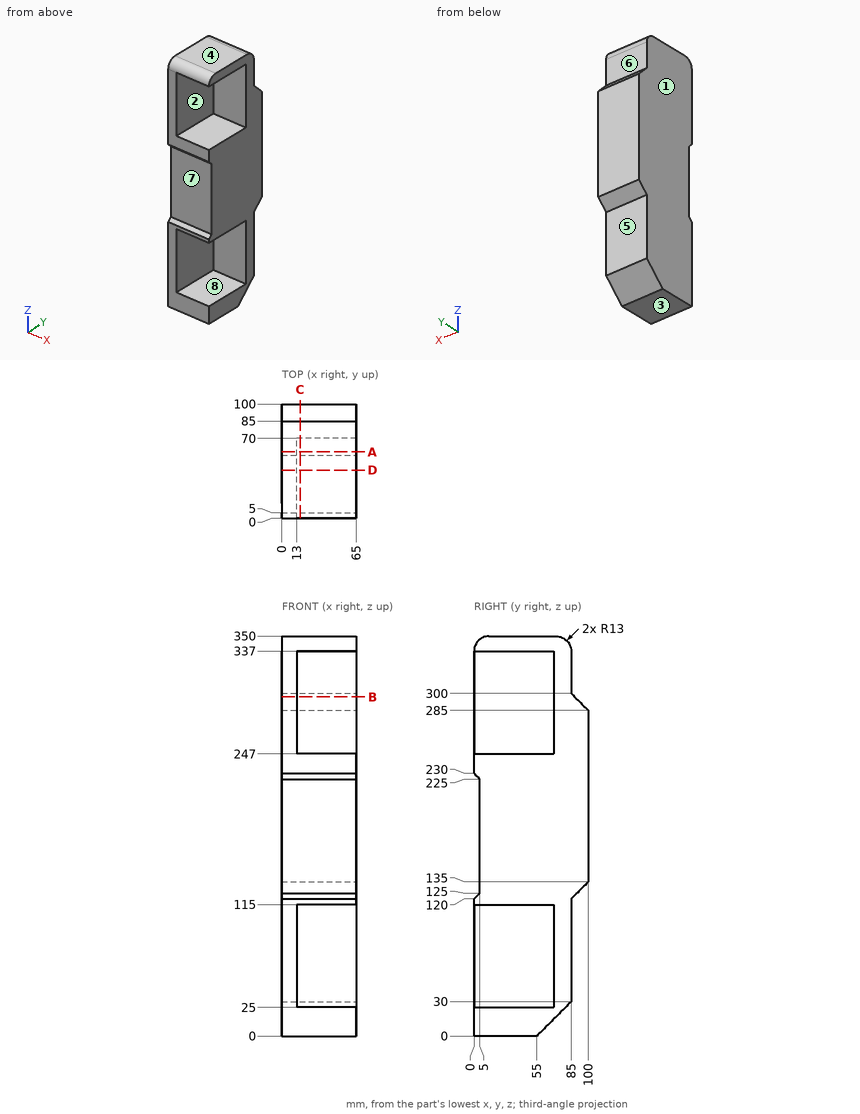
Verification items for this drawing (mm, ordinates from the low corner). A direction names the side the tool comes from. Coordinates: 2 decimals unless noted, no trailing zeros. Write each loop counter-clockwise with the first axis right and the second up, starting at its lowest first coordinate (ties: lowest second). Pieces come first, ordered by that corner, then holes. Notation, with made-up numbers: M -16,68 L 7,68 A15 cw 7,79 Z; hole C 10.5,-2.5 d9. An arc over 180 degrees is marked long. Use one line per item in the form item = value. Start each with the question number.
1) Release check for a two-part mould opening along Z. For the marked faces 1, 2, 3 and 4 record: pulls with the +Z half, pulls with the -Z half, needs draft (parallel to the pull), parting line crosses it, or undercut.
2) Section check C-C on x = 16. Enter the section's corners in (y, z), and give its area (3 significant figures).
3) Go/stop test with flat-tipped pins: pin 1 Ø3 at (x, z) = (50.5, 301) entering from +Y; pin 2 Ø19.5 at (x, z) = (26.5, 77.5) entering from +Y; pin 3 Ø15.5 at (x, z) = (40, 273.5) entering from -Y. Record where each tip stops, or that it passes through.
4) Section check D-D on y = 42. Enter the section's corners in (x, z).
5) Section check A-A on y = 58. Enter the section's corners in (x, z).
6) Thickness scan on probe 1 along Z at (x, y) = (46, 15); probe 2 along Z at (x, y) = (35, 63); probe 3 along Y at (x, z) = (40.5, 60.5). Record the ranges inside material, lowest first. Write a range as from..to.
7) Section check B-B on z = 297. Enter the section's corners in (x, y), and give its area (3 significant figures).
8) Set-up check for the marked faces 5, 6, 7 and 8: record each of +Z, -Z, +X, -X, +Y, -Y from which the full face is reachable in a straight line by a thin tool's end or side.
Responses:
q1.face_1 = needs draft
q1.face_2 = undercut
q1.face_3 = pulls with the -Z half
q1.face_4 = pulls with the +Z half
q2.outline = M 0,0 L 55,0 L 85,30 L 85,120 L 100,135 L 100,285 L 85,300 L 85,337 A13 ccw 72,350 L 13,350 A13 ccw 0,337 L 70,337 L 70,247 L 0,247 L 0,230 L 5,225 L 5,125 L 0,120 L 0,115 L 70,115 L 70,25 L 0,25 Z
q2.area = 18,600 mm2
q3.pin_1 = 85.5
q3.pin_2 = 85
q3.pin_3 = 70
q4.outline = M 0,0 L 65,0 L 65,25 L 13,25 L 13,115 L 65,115 L 65,247 L 13,247 L 13,337 L 65,337 L 65,350 L 0,350 Z
q5.outline = M 0,3 L 65,3 L 65,25 L 13,25 L 13,115 L 65,115 L 65,247 L 13,247 L 13,337 L 65,337 L 65,350 L 0,350 Z
q6.probe_1 = 0..25, 115..247, 337..350
q6.probe_2 = 8..25, 115..247, 337..350
q6.probe_3 = 70..85
q7.outline = M 0,0 L 13,0 L 13,70 L 65,70 L 65,88 L 0,88 Z
q7.area = 2,080 mm2
q8.face_5 = -Z, +X, -X, +Y
q8.face_6 = +Z, +X, -X, +Y
q8.face_7 = +X, -X, -Y
q8.face_8 = +X, -Y
